Geometry check sheet. Reference: the model listing, model coordinates, mm. A direction names the side the tool comes from. Round coordinates to 2 decimals unless told otherwise and drop trailing zeros. Loops run counter-clockwise (first coordinate to the right, second up) from the corner with the lowest first, then second, coordinate; pieces in that order, holes last. Notation, with made-up numbers: M 12,80 L 41,80 A21 ccw 41,95 Z; hole C -21.75,28 d9. An arc over 180 degrees is marked long. Use one line per item in the form item = value. Start each with the question number.
1. Set-up check for faces 1 (the flat face through (5, -66, 35)), 2 (the flat face through (0, -28, 13)): record each of +Z, -Z, +X, -X, +Y, -Y from which the full face is reachable in a straight line by a thin tool's end or side.
2. Cross-section at D-D (z = 17). Record the boundary of the cut face in (x, y).
3. Cross-section at A-A (y = -34). Record the boundary of the cut face in (x, z), then the cut area to 3 significant figures.
4. Material ranges on line 1 (Y direction, x = -8, z = 18); line 2 (Y direction, x = 1, z = 27); line 3 (Z direction, x = -0.5, y = -14), recorded low to high.
5. Go/stop test with flat-tipped pins: pin 1 (4.5 mm diameter, centred on x = 9.9, y = -10.1, fed in from +Z); pin 2 (2.5 mm diameter, centred on x = -14, y = -20, fed in from -Z); pin 3 (8 mm diameter, centred on x = 15, y = -46.5, fed in from -Z); pin 4 (9 mm diameter, centred on x = 1.5, y = -81, fed in from -Z). Record where each tip stops, or that it passes through.
6. Draft check along Z on faces 3 (the cylindrical face through (-0.195, -60.513, 33.479)), 4 (the flat face through (-6.5, -81.5, 32)), 5 (the cylindrical face through (-0.28, -59.674, 13.566)), 6 (the flat face through (0, -92, 33)). Enter one of: pulls with the +Z half, pulls with the -Z half, needs draft (parallel to the pull), parting line crosses it, or undercut.
7. Cross-section at C-C (x = -6). Record the boundary of the cut face in (y, z).
8. Cross-section at B-B (z = 3). State how many separate pieces and enclosed holes the cut face has, then the cut area to 3 significant figures.
```python
from build123d import *

# Parameters (mm, degrees)
ESQUISSE1_R           = 15
ESQUISSE1_R_2         = 5
ESQUISSE1_R_3         = 2
EXTRUSION1_DEPTH      = 13
ESQUISSE2_R           = 9
ESQUISSE2_R_2         = 1.5
EXTRUSION2_DEPTH      = 22
ESQUISSE3_R           = 15
EXTRUSION3_DEPTH      = 19
EXTRUSION4_DEPTH      = 21
EXTRUSION4_DEPTH_BACK = 21
EXTRUSION5_REACH      = 42
ESQUISSE5_R           = 2


with BuildPart() as part:
    # Esquisse1 → Extrusion1 (new body)
    with BuildSketch(Plane.XY):
        with BuildLine():
            Line((20, -20), (20, -75))
            ThreePointArc((20, -75), (0, -95), (-20, -75))
            Line((-20, -75), (-20, -20))
            ThreePointArc((-20, -20), (0, 0), (20, -20))
        make_face()
        with Locations((0, -75)):
            Circle(ESQUISSE1_R, mode=Mode.SUBTRACT)
        with Locations((0, -20)):
            Circle(ESQUISSE1_R_2, mode=Mode.SUBTRACT)
        with Locations((-14, -20)):
            Circle(ESQUISSE1_R_3, mode=Mode.SUBTRACT)
        with Locations((-9.899494937, -10.100505063)):
            Circle(ESQUISSE1_R_3, mode=Mode.SUBTRACT)
        with Locations((0, -6)):
            Circle(ESQUISSE1_R_3, mode=Mode.SUBTRACT)
        with Locations((9.899494937, -10.100505063)):
            Circle(ESQUISSE1_R_3, mode=Mode.SUBTRACT)
        with Locations((14, -20)):
            Circle(ESQUISSE1_R_3, mode=Mode.SUBTRACT)
        with Locations((9.899494937, -29.899494937)):
            Circle(ESQUISSE1_R_3, mode=Mode.SUBTRACT)
        with Locations((0, -34)):
            Circle(ESQUISSE1_R_3, mode=Mode.SUBTRACT)
        with Locations((-9.899494937, -29.899494937)):
            Circle(ESQUISSE1_R_3, mode=Mode.SUBTRACT)
    extrude(amount=EXTRUSION1_DEPTH)

    # Esquisse2 → Extrusion2 (add)
    with BuildSketch(Plane.XY.offset(13)):
        with BuildLine():
            Line((-20, -75), (-20, -51.721443851))
            ThreePointArc((-20, -51.721443851), (0, -57.5), (20, -51.721443851))
            Line((20, -51.721443851), (20, -75))
            ThreePointArc((20, -75), (0, -95), (-20, -75))
        make_face()
        with Locations((0, -75)):
            Circle(ESQUISSE2_R, mode=Mode.SUBTRACT)
        with Locations((0, -62)):
            Circle(ESQUISSE2_R_2, mode=Mode.SUBTRACT)
        with Locations((0, -88)):
            Circle(ESQUISSE2_R_2, mode=Mode.SUBTRACT)
        with Locations((-13, -75)):
            Circle(ESQUISSE2_R_2, mode=Mode.SUBTRACT)
        with Locations((13, -75)):
            Circle(ESQUISSE2_R_2, mode=Mode.SUBTRACT)
    extrude(amount=EXTRUSION2_DEPTH)

    # Esquisse3 → Extrusion3 (cut)
    with BuildSketch(Plane(origin=(0, 0, 13), x_dir=(-1, 0, 0), z_dir=(0, 0, -1))):
        with Locations((0, -75)):
            Circle(ESQUISSE3_R)
    extrude(amount=-EXTRUSION3_DEPTH, mode=Mode.SUBTRACT)

    # Esquisse4 → Extrusion4 (cut, two sides)
    with BuildSketch(Plane(origin=(0, 0, 0), x_dir=(0, 0, -1), z_dir=(1, 0, 0))) as extrusion4_sk:
        Polygon((-35, -95), (-30, -95), (-35, -90), align=None)
    extrude(amount=EXTRUSION4_DEPTH, mode=Mode.SUBTRACT)
    extrude(extrusion4_sk.sketch, amount=-EXTRUSION4_DEPTH_BACK, mode=Mode.SUBTRACT)

    # Esquisse5 → Extrusion5 (cut, up to next)
    with BuildSketch(Plane.ZY.offset(20), mode=Mode.PRIVATE) as extrusion5_sk1:
        with Locations((14, -57.721443851)):
            Circle(ESQUISSE5_R)
    extrusion5_tool1 = extrude(extrusion5_sk1.sketch, amount=-EXTRUSION5_REACH, mode=Mode.PRIVATE) & part.part
    add(extrusion5_tool1.solids().sort_by_distance((-20, -57.721444, 14))[0], mode=Mode.SUBTRACT)
    # Esquisse5 → Extrusion5 (cut, up to next)
    with BuildSketch(Plane.ZY.offset(20), mode=Mode.PRIVATE) as extrusion5_sk2:
        with Locations((3, -57.721443851)):
            Circle(ESQUISSE5_R)
    extrusion5_tool2 = extrude(extrusion5_sk2.sketch, amount=-EXTRUSION5_REACH, mode=Mode.PRIVATE) & part.part
    add(extrusion5_tool2.solids().sort_by_distance((-20, -57.721444, 3))[0], mode=Mode.SUBTRACT)


solid = part.part
```
Reported:
q1.face_1 = +Z, +X, -X, +Y, -Y
q1.face_2 = +Z, +Y
q2.outline = M -20,-75 A20 ccw 20,-75 L 20,-51.72 A37.5 cw -20,-51.72 Z; hole C 0,-75 d30
q3.outline = M -20,0 L -2,0 L -2,13 L -20,13 Z; M 2,0 L 20,0 L 20,13 L 2,13 Z
q3.area = 468 mm²
q4.line_1 = -93.33 to -87.69, -62.31 to -56.64
q4.line_2 = -94.97 to -89.97, -60.03 to -57.49
q4.line_3 = 0 to 13
q5.pin_1 = 13
q5.pin_2 = through
q5.pin_3 = 0
q5.pin_4 = 32
q6.face_3 = needs draft
q6.face_4 = pulls with the -Z half
q6.face_5 = undercut
q6.face_6 = pulls with the +Z half
q7.outline = M -94.08,0 L -88.75,0 L -88.75,32 L -81.71,32 L -81.71,35 L -90,35 L -94.08,30.92 Z; M -68.29,32 L -61.25,32 L -61.25,0 L -0.92,0 L -0.92,13 L -55.99,13 A2 cw long -57.02,15.87 L -57.02,35 L -68.29,35 Z; hole C -57.72,3 d4
q8.separate_pieces = 2
q8.enclosed_holes = 10
q8.area = 2,410 mm²
